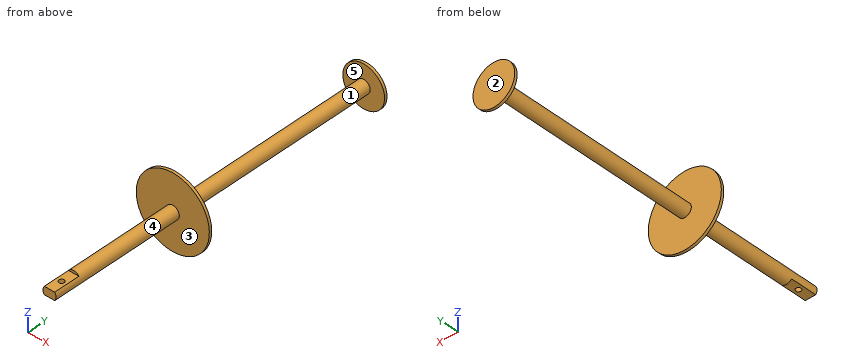
```python
from build123d import *

# Parameters (mm, degrees)
SKETCH_1_R          = 8
EXTRUDE_1_DEPTH     = 1
SKETCH_3_R          = 2.5
EXTRUDE_2_DEPTH     = 130
SKETCH_5_W          = 1
SKETCH_5_H          = 10
CUT_EXTRUDE_1_DEPTH = 131.668473627
SKETCH_6_R          = 1
CUT_EXTRUDE_2_DEPTH = 131.591921649
SKETCH_8_R          = 14
EXTRUDE_3_DEPTH     = 1


with BuildPart() as part:
    # 草图1 → 凸台-拉伸1 (new body)
    with BuildSketch(Plane(origin=(0, 0, 0), x_dir=(1, 0, 0), z_dir=(0, 1, 0))):
        with Locations(Location((0, 0, 0), (0, 0, 270))):
            Circle(SKETCH_1_R)
    extrude(amount=EXTRUDE_1_DEPTH)

    # 草图3 → 凸台-拉伸2 (add)
    with BuildSketch(Plane.XZ):
        with Locations(Location((0, 0, 0), (0, 0, 270))):
            Circle(SKETCH_3_R)
    extrude(amount=EXTRUDE_2_DEPTH)

    # 草图5 → 切除-拉伸1 (cut, through all)
    with BuildSketch(Plane(origin=(2.5, 0, 0), x_dir=(0, 0, -1), z_dir=(1, 0, 0))):
        with Locations((-2, -125)):
            Rectangle(SKETCH_5_W, SKETCH_5_H)
        with Locations((2, -125)):
            Rectangle(SKETCH_5_W, SKETCH_5_H)
    extrude(amount=-CUT_EXTRUDE_1_DEPTH, mode=Mode.SUBTRACT)

    # 草图6 → 切除-拉伸2 (cut, through all)
    with BuildSketch(Plane.XY.offset(1.5)):
        with Locations((0, -125)):
            Circle(SKETCH_6_R)
    extrude(amount=-CUT_EXTRUDE_2_DEPTH, mode=Mode.SUBTRACT)

    # 草图8 → 凸台-拉伸3 (add)
    with BuildSketch(Plane(origin=(0, -79, 0), x_dir=(1, 0, 0), z_dir=(0, 1, 0))):
        with Locations(Location((0, 0, 0), (0, 0, 270))):
            Circle(SKETCH_8_R)
    extrude(amount=EXTRUDE_3_DEPTH)


solid = part.part
```
Here's how the part is built. I have some questions about the finished solid (model axes, mm). Face numbers are marked on the shaded views. A direction names the side the tool comes from. Give positions to 0.01 mm unless a question says otherwise; leave off trailing zeros. Write each loop counter-clockwise with the first axis right and the second up, starting at its lowest first coordinate (ties: lowest second). Pieces come first, ordered by that corner, then holes.
(1) Will these pins go through, and if not, where does the flat tip stop? pin 1 (0.5 mm diameter, centred on x = -0.5, z = 2, fed in from -Y); pin 2 (5 mm diameter, centred on x = 11, z = -5, fed in from +Y); pin 3 (12 mm diameter, centred on y = -83.5, z = 7.5, fed in from +X); pin 4 (1.2 mm diameter, centred on x = 0, y = -125, fed in from -Z).
Output values:
pin 1: stops at y = -120
pin 2: stops at y = -78
pin 3: stops at x = 13.55
pin 4: passes through
(2) Imagine slicing it at D-D, the plane x = 11.25. Write out the boundary of the cut face in (y, z), and give its area (3 significant figures).
Output values:
outline: (-79, -8.33) - (-78, -8.33) - (-78, 8.33) - (-79, 8.33) - close
area: 16.7 mm2
(3) Imagine slicing it at C-C, the plane y = -110. Write out the boundary of the cut face in (x, z), and give its area (3 significant figures).
Output values:
outline: circle Ø5 at (0, 0)
area: 19.6 mm2
(4) Thinking about a two-plate mould opening in Y: for the marked faces 3, 4 and 5, which applies, pulls with the +Y half, pulls with the -Y half, needs draft (parallel to the pull), parting line crosses it, or undercut?
Output values:
face 3: pulls with the -Y half
face 4: needs draft
face 5: undercut
(5) On a 3-axis mill with a long thin cutter (end or side, diameter ignored), from which of +Z, -Z, +X, -X, +Y, -Y can I reach the whole of each face in a straight line? I mean the marked faces 1 and 2. Say none if no direction works.
Output values:
face 1: none
face 2: +Z, -Z, +X, -X, +Y
(6) Imagine slicing it at A-A, the plane z = 0. Write out the boundary of the cut face in (x, y), and give its area (3 significant figures).
Output values:
outline: (-14, -79) - (-2.5, -79) - (-2.5, -130) - (2.5, -130) - (2.5, -79) - (14, -79) - (14, -78) - (2.5, -78) - (2.5, 0) - (8, 0) - (8, 1) - (-8, 1) - (-8, 0) - (-2.5, 0) - (-2.5, -78) - (-14, -78) - close; hole circle Ø2 at (0, -125)
area: 686 mm2
(7) Imagine slicing it at B-B, the plane z = 5.5. Write out the boundary of the cut face in (x, y).
Output values:
outline: (-12.87, -79) - (12.87, -79) - (12.87, -78) - (-12.87, -78) - close; (-5.81, 0) - (5.81, 0) - (5.81, 1) - (-5.81, 1) - close
(8) If I drill on L1, parallel to Y at x = -0.75, z = -2.5; L2, parallel to X at y = -125, z = -0.35; L3, parallel to Y at x = -10.5, z = -6, over which ranges is the centre line in solid material (lowest first)?
Output values:
L1: y = -79 to -78, 0 to 1
L2: x = -2.48 to -1, 1 to 2.48
L3: y = -79 to -78
